from build123d import *

# Parameters (mm, degrees)
EXTRUDE_1_DEPTH     = 15
SKETCH_2_R          = 3.1
CUT_EXTRUDE_1_DEPTH = 12
CUT_EXTRUDE_START   = -7.5
CUT_EXTRUDE_2_DEPTH = 7.5
SKETCH_4_R          = 1.6
CUT_EXTRUDE_3_DEPTH = 8
CUT_EXTRUDE_4_DEPTH = 3
FILLET_1_R          = 3


with BuildPart() as part:
    # Model → 凸台-拉伸1 (new body)
    with BuildSketch(Plane.XY):
        with BuildLine():
            Line((113.596149123, 231.939716908), (128.596149123, 231.939716908))
            Line((128.596149123, 231.939716908), (128.596149123, 270.519406691))
            ThreePointArc((128.596149123, 270.519406691), (129.205112863, 273.58087415), (130.939294874, 276.17626094))
            Line((130.939294874, 276.17626094), (158.219255135, 303.456221202))
            ThreePointArc((158.219255135, 303.456221202), (158.219255135, 314.06282292), (147.612653418, 314.06282292))
            Line((147.612653418, 314.06282292), (115.939294874, 282.389464376))
            ThreePointArc((115.939294874, 282.389464376), (114.205112863, 279.794077585), (113.596149123, 276.732610126))
            Line((113.596149123, 276.732610126), (113.596149123, 231.939716908))
        make_face()
    extrude(amount=EXTRUDE_1_DEPTH)

    # 草图2 → 切除-拉伸1 (cut)
    with BuildSketch(Plane.XZ.offset(-231.939716908)):
        with Locations(Location((121.096149123, 7.5, 0), (0, 0, 270))):
            Circle(SKETCH_2_R)
    extrude(amount=-CUT_EXTRUDE_1_DEPTH, mode=Mode.SUBTRACT)

    # 草图3 → 切除-拉伸2 (cut)
    with BuildSketch(Plane.XY.offset(15).offset(CUT_EXTRUDE_START)):
        with BuildLine():
            Line((114.205112863, 279.794077585), (129.205112863, 273.58087415))
            ThreePointArc((129.205112863, 273.58087415), (129.944392225, 274.963968555), (130.939294874, 276.17626094))
            Line((130.939294874, 276.17626094), (158.219255135, 303.456221202))
            ThreePointArc((158.219255135, 303.456221202), (158.219255135, 314.06282292), (147.612653418, 314.06282292))
            Line((147.612653418, 314.06282292), (115.939294874, 282.389464376))
            ThreePointArc((115.939294874, 282.389464376), (114.944392225, 281.17717199), (114.205112863, 279.794077585))
        make_face()
    extrude(amount=CUT_EXTRUDE_2_DEPTH, mode=Mode.SUBTRACT)

    # 草图4 → 切除-拉伸3 (cut)
    with BuildSketch(Plane.XY.offset(7.5)):
        with Locations((152.915954276, 308.759522061)):
            Circle(SKETCH_4_R)
    extrude(amount=-CUT_EXTRUDE_3_DEPTH, mode=Mode.SUBTRACT)

    # 草图5 → 切除-拉伸4 (cut)
    with BuildSketch(Plane(origin=(0, 0, 0), x_dir=(-1, 0, 0), z_dir=(0, 0, -1))):
        Polygon((-149.682792769, 308.759522061), (-151.299373523, 311.559522061), (-154.53253503, 311.559522061), (-156.149115784, 308.759522061), (-154.53253503, 305.959522061), (-151.299373523, 305.959522061), align=None)
    extrude(amount=-CUT_EXTRUDE_4_DEPTH, mode=Mode.SUBTRACT)

    # 圆角1
    # the kernel refuses this fillet: 3 mm, written as the material it takes off along each edge
    with BuildSketch(Plane(origin=(113.596149123, 276.732610126, 0), x_dir=(0, 0, 1), z_dir=(0, -1, 0))) as fillet_1_piece_1:
        with BuildLine():
            CenterArc((FILLET_1_R, -FILLET_1_R), FILLET_1_R, 90, 90)
            Line((0, -FILLET_1_R), (0, 0))
            Line((0, 0), (FILLET_1_R, 0))
        make_face()
    extrude(amount=52.292893219, mode=Mode.SUBTRACT)
    with BuildSketch(Plane(origin=(121.596149123, 276.732610126, 0), x_dir=(-0.7071067811865422, 0.7071067811865529, 0), z_dir=(0.7071067811865529, 0.7071067811865422, 0))) as fillet_1_piece_2:
        with BuildLine():
            CenterArc((8 - FILLET_1_R, FILLET_1_R), FILLET_1_R, 270, 90)
            Line((8, FILLET_1_R), (8, 0))
            Line((8, 0), (8 - FILLET_1_R, 0))
        make_face()
    revolve(axis=Axis((121.596149123, 276.732610126, 0), (0, 0, 1)), revolution_arc=45, mode=Mode.SUBTRACT)
    with BuildSketch(Plane(origin=(147.612653418, 314.06282292, 0), x_dir=(0.7071067811865483, -0.7071067811865468, 0), z_dir=(-0.7071067811865469, -0.7071067811865482, 0))) as fillet_1_piece_3:
        with BuildLine():
            CenterArc((FILLET_1_R, FILLET_1_R), FILLET_1_R, 180, 90)
            Line((0, FILLET_1_R), (0, 0))
            Line((0, 0), (FILLET_1_R, 0))
        make_face()
    extrude(amount=44.792893219, mode=Mode.SUBTRACT)
    with BuildSketch(Plane(origin=(152.915954276, 308.759522061, 0), x_dir=(0.7071067811865419, -0.7071067811865532, 0), z_dir=(-0.7071067811865532, -0.7071067811865419, 0))) as fillet_1_piece_4:
        with BuildLine():
            CenterArc((7.5 - FILLET_1_R, FILLET_1_R), FILLET_1_R, 270, 90)
            Line((7.5, FILLET_1_R), (7.5, 0))
            Line((7.5, 0), (7.5 - FILLET_1_R, 0))
        make_face()
    revolve(axis=Axis((152.915954276, 308.759522061, 0), (0, 0, 1)), revolution_arc=180, mode=Mode.SUBTRACT)
    with BuildSketch(Plane(origin=(130.939294874, 276.17626094, 0), x_dir=(-0.707106781186548, 0.7071067811865471, 0), z_dir=(0.7071067811865471, 0.7071067811865479, 0))) as fillet_1_piece_5:
        with BuildLine():
            CenterArc((FILLET_1_R, FILLET_1_R), FILLET_1_R, 180, 90)
            Line((0, FILLET_1_R), (0, 0))
            Line((0, 0), (FILLET_1_R, 0))
        make_face()
    extrude(amount=38.579689783, mode=Mode.SUBTRACT)
    with BuildSketch(Plane(origin=(136.596149123, 270.519406691, 0), x_dir=(-1, 0, 0), z_dir=(0, -1, 0))) as fillet_1_piece_6:
        with BuildLine():
            CenterArc((8 + FILLET_1_R, -FILLET_1_R), FILLET_1_R, 90, 90)
            Line((8, -FILLET_1_R), (8, 0))
            Line((8, 0), (8 + FILLET_1_R, 0))
        make_face()
    revolve(axis=Axis((136.596149123, 270.519406691, 0), (0, 0, -1)), revolution_arc=45, mode=Mode.SUBTRACT)
    with BuildSketch(Plane(origin=(136.596149123, 270.519406691, 15), x_dir=(-1, 0, 0), z_dir=(0, -1, 0))) as fillet_1_piece_7:
        with BuildLine():
            CenterArc((8 + FILLET_1_R, FILLET_1_R), FILLET_1_R, 180, 90)
            Line((8, FILLET_1_R), (8, 0))
            Line((8, 0), (8 + FILLET_1_R, 0))
        make_face()
    revolve(axis=Axis((136.596149123, 270.519406691, 15), (0, 0, -1)), revolution_arc=76.216141543, mode=Mode.SUBTRACT)
    with BuildSketch(Plane(origin=(128.596149123, 224.439716908, 0), x_dir=(-1, 0, 0), z_dir=(0, 1, 0))) as fillet_1_piece_8:
        with BuildLine():
            CenterArc((FILLET_1_R, FILLET_1_R), FILLET_1_R, 180, 90)
            Line((0, FILLET_1_R), (0, 0))
            Line((0, 0), (FILLET_1_R, 0))
        make_face()
    extrude(amount=46.079689783, mode=Mode.SUBTRACT)
    with BuildSketch(Plane(origin=(128.596149123, 224.439716908, 15), x_dir=(-1, 0, 0), z_dir=(0, 1, 0))) as fillet_1_piece_9:
        with BuildLine():
            CenterArc((FILLET_1_R, -FILLET_1_R), FILLET_1_R, 90, 90)
            Line((0, -FILLET_1_R), (0, 0))
            Line((0, 0), (FILLET_1_R, 0))
        make_face()
    extrude(amount=46.079689783, mode=Mode.SUBTRACT)
    with BuildSketch(Plane(origin=(107.276016369, 282.664203328, 15), x_dir=(-0.38268343236508984, -0.9238795325112866, 0), z_dir=(0.9238795325112867, -0.38268343236508984, 0))) as fillet_1_piece_10:
        with BuildLine():
            CenterArc((FILLET_1_R, FILLET_1_R), FILLET_1_R, 180, 90)
            Line((0, FILLET_1_R), (0, 0))
            Line((0, 0), (FILLET_1_R, 0))
        make_face()
    extrude(amount=31.235883004, mode=Mode.SUBTRACT)
    with BuildSketch(Plane(origin=(113.596149123, 276.732610126, 15), x_dir=(0, 0, -1), z_dir=(0, -1, 0))) as fillet_1_piece_11:
        with BuildLine():
            CenterArc((FILLET_1_R, FILLET_1_R), FILLET_1_R, 180, 90)
            Line((0, FILLET_1_R), (0, 0))
            Line((0, 0), (FILLET_1_R, 0))
        make_face()
    extrude(amount=52.292893219, mode=Mode.SUBTRACT)
    with BuildSketch(Plane(origin=(121.596149123, 276.732610126, 15), x_dir=(-0.23825985719225534, 0.9712014417466266, 0), z_dir=(0.9712014417466266, 0.23825985719225534, 0))) as fillet_1_piece_12:
        with BuildLine():
            CenterArc((8 - FILLET_1_R, -FILLET_1_R), FILLET_1_R, 0, 90)
            Line((8, -FILLET_1_R), (8, 0))
            Line((8, 0), (8 - FILLET_1_R, 0))
        make_face()
    revolve(axis=Axis((121.596149123, 276.732610126, 15), (0, 0, 1)), revolution_arc=76.216141543, mode=Mode.SUBTRACT)


solid = part.part
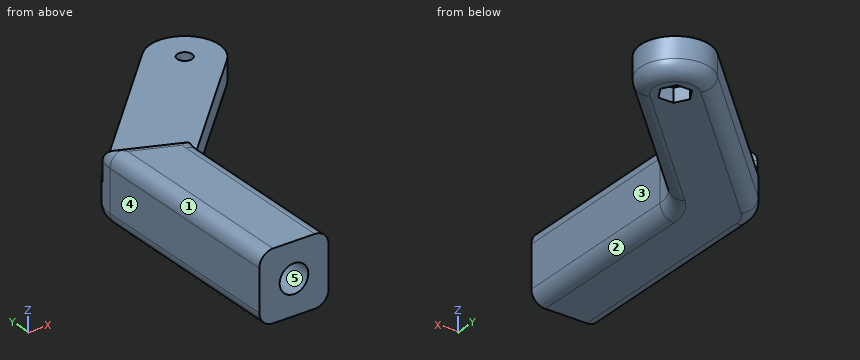
The model under review builds one solid part; all positions refer to its coordinate system, in mm. Face numbers are marked on the shaded views. A direction names the side the tool comes from. Coordinates: 2 decimals unless noted, no trailing zeros. Loops run counter-clockwise (first coordinate to the right, second up) from the corner with the lowest first, then second, coordinate; pieces in that order, holes last. Notation, with made-up numbers: (-2, -33) -> (50, -33) arc R25 cw to (50, -9) -> close; hole circle Ø2 at (30, 54.25). An arc over 180 degrees is marked (long way). Use a Markdown table: item, result. Add a question column.
1. Add section B-B on y = 239. Write out the cut boundary in (x, z).
2. Add section C-C on z = 9.25. Write out the cut boundary in (x, y).
3. To check wall thickness, follow line 1 (X direction, y = 240.75, z = 7.5); line 2 (X direction, y = 244, z = 4.5); line 3 (Z direction, x = 129.5, y = 285). State the ranges of each line that lie inside material, in increasing order.
4. Add section A-A on y = 255. Write out the cut boundary in (x, z).
5. Draft analysis for pull direction X (two halves, no side actions). For the marked faces 3, 4 and 5, state which applies: pulls with the +X half, pulls with the -X half, needs draft (parallel to the pull), parting line crosses it, or undercut.
6. Clearance check with flat-ended pins moving along their axes: pin 1 Ø8 at (y, z) = (281.5, 11.5) entering from -X; pin 2 Ø3 at (y, z) = (277.5, 5) entering from +X; pin 3 Ø4 at (x, y) = (130.5, 288.5) entering from +Z; pin 4 Ø3 at (x, y) = (152.92, 308.76) entering from +Z. State where each tip first meets the part, or that it passes through.
7. Machinability: for the marked faces 1 and 2, which of the approach directions +Z, -Z, +X, -X, +Y, -Y give a long, thin tool a straight path to every point of the face, cutting with its end or side? Answer none if there is none.
Returned:
| question | item | result |
|---|---|---|
| 1 | outline | (113.6, 3) arc R3 ccw to (116.6, 0) -> (125.6, 0) arc R3 ccw to (128.6, 3) -> (128.6, 12) arc R3 ccw to (125.6, 15) -> (116.6, 15) arc R3 ccw to (113.6, 12) -> close; hole circle Ø6.2 at (121.1, 7.5) |
| 2 | outline | (113.6, 231.94) -> (118.54, 231.94) -> (118.54, 243.94) -> (123.65, 243.94) -> (123.65, 231.94) -> (128.6, 231.94) -> (128.6, 270.52) arc R8 cw to (129.21, 273.58) -> (114.21, 279.79) arc R8 ccw to (113.6, 276.73) -> close |
| 3 | line 1 | x = 113.6 to 118, 124.2 to 128.6 |
| 3 | line 2 | x = 113.6 to 128.6 |
| 3 | line 3 | z = 0 to 7.5 |
| 4 | outline | (113.6, 3) arc R3 ccw to (116.6, 0) -> (125.6, 0) arc R3 ccw to (128.6, 3) -> (128.6, 12) arc R3 ccw to (125.6, 15) -> (116.6, 15) arc R3 ccw to (113.6, 12) -> close |
| 5 | face 3 | pulls with the +X half |
| 5 | face 4 | pulls with the -X half |
| 5 | face 5 | undercut |
| 6 | pin 1 | stops at x = 113.63 |
| 6 | pin 2 | stops at x = 133.76 |
| 6 | pin 3 | stops at z = 7.5 |
| 6 | pin 4 | passes through |
| 7 | face 1 | +Z, -X, +Y, -Y |
| 7 | face 2 | -Z, +X, -Y |
